Geometry: see drawing. Coordinates: mm, zero at the bounding-box minimum. A direction names the side the tool comes from. Round coordinates to 2 decimals unless told otherwise and drop trailing zeros. Loops run counter-clockwise (first coordinate to the right, second up) from the corner with the lowest first, then second, coordinate; pieces in that order, holes last. Notation, with made-up numbers: (87, 87.25) - (125, 87.25) arc R17 cw to (125, 107.25) - close; hole circle Ø3 at (36.5, -23). An arc over 180 degrees is marked (long way). Use CSV: the item, a comma, the result in double quotes. Start each with the question number.
1. Cut plane D-D (z = 2). Return loops of the section in (x, y), and give its area (3 significant figures).
2. Pin query (flat end, axial travel): P1, Ø5, axis at x = 8, z = 1.5, coming from the +Y side; P2, Ø1.5, axis at y = 10.5, z = 4, coming from the +X side; P3, Ø5, axis at y = 3.5, z = 7, coming from the -X side. Return the tip coordinate at first contact, or that it passes through.
3. Cut plane C-C (z = 5.5). Return loops of the section in (x, y) (3 decimals).
4. Pull-direction query (X, two-part tool) for the marked faces 3, 4 and 5; classes: +X half, -X half, draft (parallel to the pull), parting line (faces both ways), or undercut.
5. Material intervals for probe 1 along X at (y, z) = (19.5, 7.5); probe 2 along Z at (x, y) = (16, 37); probe 3 along Y at (x, z) = (20, 3.75), sorted ascending. Write a range as from..to.
6. Access query for the marked faces 1 and 2. Directions: +Z, -Z, +X, -X, +Y, -Y. A direction counts if a zero-diameter tool reaches every point of the face in a straight line with its end or side. Return the directions, or none.
7. Cut plane A-A (y = 20). Return loops of the section in (x, z).
8. Cut plane B-B (x = 13.5). Return loops of the section in (y, z).
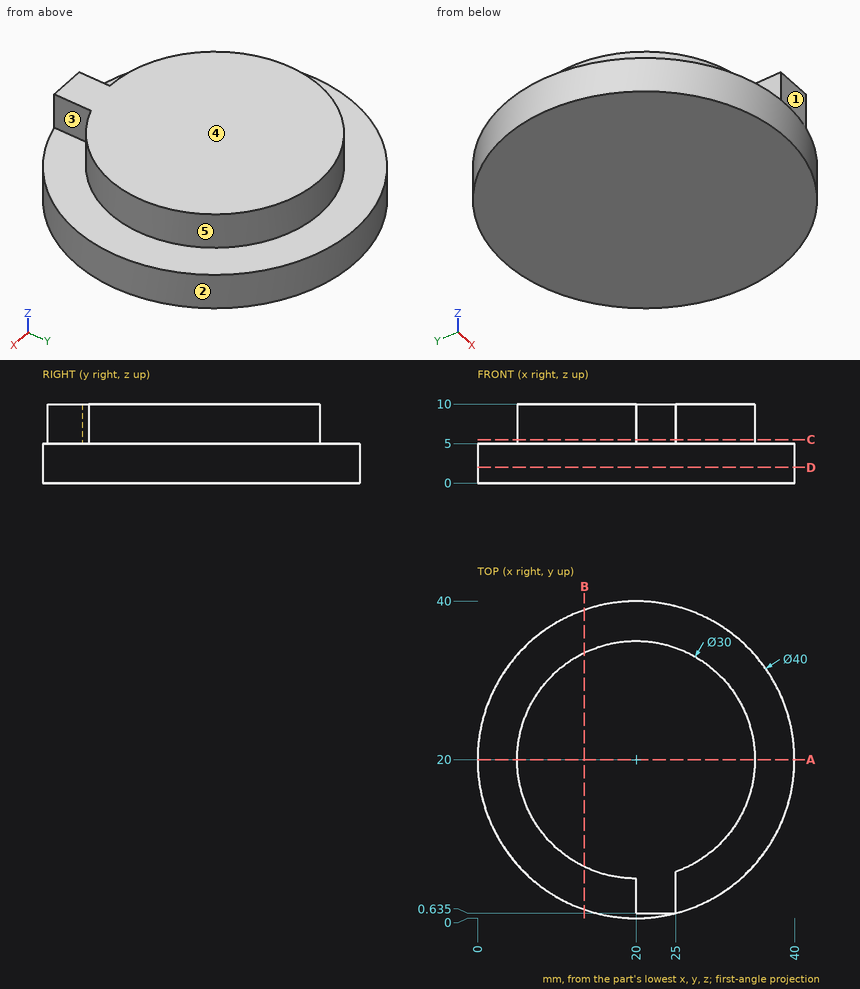
Established:
1,outline,"circle Ø40 at (20, 20)"
1,area,"1,260 mm2"
2,P1,"stops at y = 37.6"
2,P2,"stops at x = 37.98"
2,P3,"stops at x = 6.77"
3,outline,"(20, 0.635) - (25, 0.635) - (25, 5.858) arc R15 ccw (long way) to (20, 5) - close"
4,face 3,"+X half"
4,face 4,"draft"
4,face 5,"parting line"
5,probe 1,"x = 5.01..34.99"
5,probe 2,"z = 0..5"
5,probe 3,"y = 0..40"
6,face 1,"+Z, +X, -X, -Y"
6,face 2,"+Z, -Z"
7,outline,"(0, 0) - (40, 0) - (40, 5) - (35, 5) - (35, 10) - (5, 10) - (5, 5) - (0, 5) - close"
8,outline,"(1.09, 0) - (38.91, 0) - (38.91, 5) - (33.52, 5) - (33.52, 10) - (6.48, 10) - (6.48, 5) - (1.09, 5) - close"
